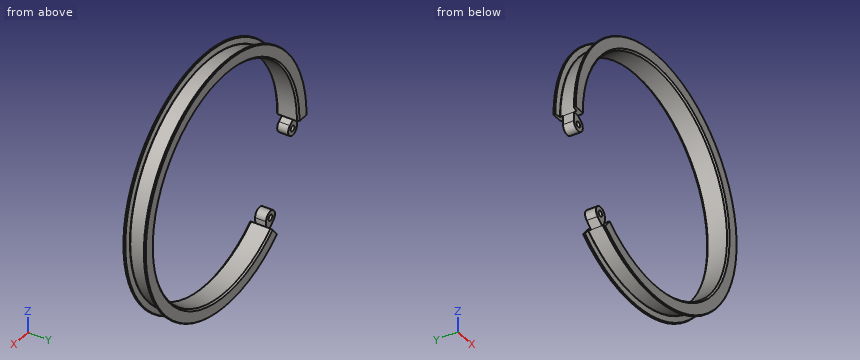
```python
from build123d import *

# Parameters (mm, degrees)
BOSS_EXTRUDE2_DEPTH      = 3.175
BOSS_EXTRUDE2_DEPTH_BACK = 3.175
SKETCH5_R                = 1.651


with BuildPart() as part:
    # Sweep2: sweep along a path in Sketch4
    with BuildLine(Plane(origin=(0, 0, 0), x_dir=(1, 0, 0), z_dir=(0, 1, 0))) as sweep2_path:
        ThreePointArc((-66.167, 0), (59.78583857, -28.350051068), (-41.873155771, 51.231930617))
    # Sketch1 → Sweep2 (sweep)
    with BuildSketch(Plane.XY):
        with BuildLine():
            Line((-68.072, 4.699), (-68.072, -4.699))
            ThreePointArc((-68.072, -4.699), (-68.117948863, -4.772140282), (-68.185476115, -4.826))
            Line((-68.185476115, -4.826), (-71.374, -5.38822279))
            Line((-71.374, -5.38822279), (-71.628, -5.64222279))
            Line((-71.628, -5.64222279), (-71.628, -6.233150289))
            Line((-71.628, -6.233150289), (-71.374, -6.487150289))
            Line((-71.374, -6.487150289), (-65.145686506, -6.487150289))
            Line((-65.145686506, -6.487150289), (-64.262, -5.603463784))
            Line((-64.262, -5.603463784), (-64.262, 5.603463784))
            Line((-64.262, 5.603463784), (-65.145686506, 6.487150289))
            Line((-65.145686506, 6.487150289), (-71.374, 6.487150289))
            Line((-71.374, 6.487150289), (-71.628, 6.233150289))
            Line((-71.628, 6.233150289), (-71.628, 5.64222279))
            Line((-71.628, 5.64222279), (-71.374, 5.38822279))
            Line((-71.374, 5.38822279), (-68.185476115, 4.826))
            ThreePointArc((-68.185476115, 4.826), (-68.117948863, 4.772140282), (-68.072, 4.699))
        make_face()
    sweep(path=sweep2_path.line)

    # Sketch5 → Boss-Extrude2 (add, two sides: drawn at the far end of the back side and taken through both)
    # profile 1 of 2: a face of its own
    with BuildSketch(Plane(origin=(0, 0, 0), x_dir=(1, 0, 0), z_dir=(0, 1, 0)).offset(-BOSS_EXTRUDE2_DEPTH_BACK)):
        with BuildLine():
            Line((-68.072, 0), (-67.997817291, 5.05529393))
            ThreePointArc((-67.997817291, 5.05529393), (-62.347816522, 8.624761173), (-61.63409996, 1.979897461))
            Line((-61.63409996, 1.979897461), (-64.262, 0))
            Line((-64.262, 0), (-68.072, 0))
        make_face()
        with Locations(Location((-64.060894811, 5.08, 0), (0, 0, 270))):
            Circle(SKETCH5_R, mode=Mode.SUBTRACT)
    # profile 2 of 2: a face of its own
    with BuildSketch(Plane(origin=(0, 0, 0), x_dir=(1, 0, 0), z_dir=(0, 1, 0)).offset(-BOSS_EXTRUDE2_DEPTH_BACK)):
        with BuildLine():
            Line((-40.533809509, 46.472492493), (-40.663586841, 49.760198444))
            Line((-40.663586841, 49.760198444), (-43.074471436, 52.710407838))
            Line((-43.074471436, 52.710407838), (-46.942012037, 49.454086372))
            ThreePointArc((-46.942012037, 49.454086372), (-46.130772136, 42.82042261), (-40.533809509, 46.472492493))
        make_face()
        with Locations(Location((-44.469944405, 46.389963231, 0), (0, 0, 90))):
            Circle(SKETCH5_R, mode=Mode.SUBTRACT)
    extrude(amount=BOSS_EXTRUDE2_DEPTH + BOSS_EXTRUDE2_DEPTH_BACK)


solid = part.part
```
The model under review builds one solid part; all positions refer to its coordinate system, in mm. Give positions to 0.01 mm unless a question says otherwise; leave off trailing zeros. Write each question's results on one line, items separated by ' | '. Start each with the question number.
1. For probe 1 along X at (y, z) = (0.75, -5.08); probe 2 along X at (y, z) = (-0.75, 0); probe 3 along X at (y, z) = (-1.5, 2), list the stretches that pass through material, from the lowest coordinate up. Write a range as [from, to].
2. We need section A-A (y = -1). Count the separate pieces of the cut face and the enclosed holes in it, and give its area (3 significant figures).
3. Insertion check: pin 1 Ø1 at (x, y) = (-67.5, 5) entering from -Z; pin 2 Ø2 at (x, y) = (0, -4.5) entering from +Z; pin 3 Ø2 at (y, z) = (0.5, 31) entering from +X; pin 4 Ø2 at (x, z) = (-64.06, -5.08) entering from +Y. Each pin has a flat end and moves straight along its axis. Give the tip position at first contact, or say it passes through.
Results found:
1) probe 1: x = [-68, -65.71], [-62.41, -60.12], [64.06, 67.88] | probe 2: x = [-68.07, -64.26], [64.26, 68.07] | probe 3: x = [-68.04, -64.23], [64.23, 68.04]
2) separate pieces: 1 | enclosed holes: 2 | area: 1,460 mm^2
3) pin 1: stops at z = 0 | pin 2: stops at z = 71.49 | pin 3: stops at x = 61.1 | pin 4: passes through
